Work out the finished part from the listing and answer in its coordinate system (mm). A direction names the side the tool comes from. Give positions to 0.01 mm unless a question says otherwise; leave off trailing zeros. Order: outer loops, then holes, each group sorted by start corner. A loop starts at its lowest first (then second) coordinate and runs counter-clockwise, first axis right, second up. Notation, with made-up numbers: (88.25, 5.25) - (107.25, 5.25) arc R22 cw to (107.25, 44.25) - close; hole circle Ø3 at (31.25, 77). An arc over 180 degrees is marked (long way). Write each question's results on one line, items separated by ' | '.
from build123d import *

# Parameters (mm, degrees)
F0_R     = 6.35
F1_DEPTH = 88.9
F2_R     = 6.35
F2_R_2   = 2.69875
F3_DEPTH = 12.7
F4_R     = 6.35
F4_R_2   = 5.08
F5_DEPTH = 12.7


with BuildPart() as f1:
    # F0 (on Top) → F1 (new body, symmetric)
    with BuildSketch(Plane.XY):
        Circle(F0_R)
    extrude(amount=F1_DEPTH, both=True)

    # F2 (on face) → F3 (cut)
    with BuildSketch(Plane.XY.offset(88.9)):
        Circle(F2_R)
        Circle(F2_R_2, mode=Mode.SUBTRACT)
    extrude(amount=-F3_DEPTH, mode=Mode.SUBTRACT)

    # F4 (on face) → F5 (cut)
    with BuildSketch(Plane(origin=(0, 0, -88.9), x_dir=(1, 0, 0), z_dir=(0, 0, -1))):
        Circle(F4_R)
        Circle(F4_R_2, mode=Mode.SUBTRACT)
    extrude(amount=-F5_DEPTH, mode=Mode.SUBTRACT)


solid = f1.part
1. A cutting plane is placed at A-A, the plane x = 0. Write down the section's boundary in (y, z).
Answer list:
outline: (-6.35, -76.2) - (-5.08, -76.2) - (-5.08, -88.9) - (5.08, -88.9) - (5.08, -76.2) - (6.35, -76.2) - (6.35, 76.2) - (2.7, 76.2) - (2.7, 88.9) - (-2.7, 88.9) - (-2.7, 76.2) - (-6.35, 76.2) - close
2. Straight lines are drawn through the part: line 1 (Z direction, x = -4, y = 2); line 2 (Z direction, x = 4, y = 3.75); line 3 (X direction, y = -5.25, z = 34.5). For each, find the intervals that lie inside material, in ascending order. Write a range as [from, to].
Answer list:
line 1: [-88.9, 76.2] | line 2: [-76.2, 76.2] | line 3: [-3.57, 3.57]
3. Given P1, Ø1.5, axis at y = 2, z = 18.5, coming from the +X side; P2, Ø5, axis at x = -3, y = 2, coming from the +Z side; P3, Ø1.5, axis at x = -4, z = -44, coming from the -Y side; P4, Ø4, axis at x = -4.5, z = 18, coming from the +Y side, each flat-ended and moving along its own axis, determine where each tip first touches the part or whether it passes through.
Answer list:
P1: x = 6.23 | P2: z = 88.9 | P3: y = -5.46 | P4: y = 5.84
4. A tool of negligible diameter and unlimited length cuts with its end or side. For faces 1 (the face through (-0.661, -5.037, -82.639)), 2 (the face through (-1.99, 1.82, 82.64)), 3 (the face through (0, 0, -88.9)), from which of +Z, -Z, +X, -X, +Y, -Y can it reach the whole face along a straight path? Write none if from no direction.
Answer list:
face 1: -Z | face 2: +Z | face 3: -Z, +X, -X, +Y, -Y
